```python
from build123d import *

# Parameters (mm, degrees)
SKETCH1_W           = 70
SKETCH1_H           = 70
SKETCH1_R           = 5
BOSS_EXTRUDE1_DEPTH = 5
SKETCH2_W           = 13.5
SKETCH2_H           = 7
SKETCH2_W_2         = 12
BOSS_EXTRUDE2_DEPTH = 20
SKETCH3_R           = 1.75
CUT_EXTRUDE1_DEPTH  = 20
SKETCH4_R           = 4
CUT_EXTRUDE2_DEPTH  = 3
BOSS_EXTRUDE3_START = 1
SKETCH5_R           = 6
SKETCH5_R_2         = 4
BOSS_EXTRUDE3_DEPTH = 1
SKETCH6_R           = 15
CUT_EXTRUDE3_DEPTH  = 83.158383626


with BuildPart() as part:
    # Sketch1 → Boss-Extrude1 (new body)
    with BuildSketch(Plane.XY):
        Rectangle(SKETCH1_W, SKETCH1_H)
        with Locations((0, -14)):
            Circle(SKETCH1_R, mode=Mode.SUBTRACT)
    extrude(amount=BOSS_EXTRUDE1_DEPTH)

    # Sketch2 → Boss-Extrude2 (add)
    with BuildSketch(Plane.XY.offset(5)):
        with Locations((-28.25, -31.5)):
            Rectangle(SKETCH2_W, SKETCH2_H)
        with Locations((28.25, -31.5)):
            Rectangle(SKETCH2_W, SKETCH2_H)
        with Locations((0, -31.5)):
            Rectangle(SKETCH2_W_2, SKETCH2_H)
    extrude(amount=BOSS_EXTRUDE2_DEPTH)

    # Sketch3 → Cut-Extrude1 (cut)
    with BuildSketch(Plane(origin=(0, -28, 0), x_dir=(1, 0, 0), z_dir=(0, 1, 0))):
        with Locations(Location((-28.25, -10, 0), (0, 0, 270))):
            Circle(SKETCH3_R)
        with Locations(Location((28.25, -10, 0), (0, 0, 270))):
            Circle(SKETCH3_R)
        with Locations(Location((0, -20, 0), (0, 0, 270))):
            Circle(SKETCH3_R)
    extrude(amount=-CUT_EXTRUDE1_DEPTH, mode=Mode.SUBTRACT)

    # Sketch4 → Cut-Extrude2 (cut)
    with BuildSketch(Plane.XY.offset(5)):
        with Locations((0, 26)):
            Circle(SKETCH4_R)
    extrude(amount=-CUT_EXTRUDE2_DEPTH, mode=Mode.SUBTRACT)

    # Sketch5 → Boss-Extrude3 (add)
    with BuildSketch(Plane.XY.offset(5).offset(BOSS_EXTRUDE3_START)):
        with Locations((0, 26)):
            Circle(SKETCH5_R)
        with Locations((0, 26)):
            Circle(SKETCH5_R_2, mode=Mode.SUBTRACT)
    extrude(amount=-BOSS_EXTRUDE3_DEPTH)

    # Sketch6 → Cut-Extrude3 (cut, through all)
    with BuildSketch(Plane.XZ.offset(35)):
        with Locations((0, 38.5)):
            Circle(SKETCH6_R)
    extrude(amount=-CUT_EXTRUDE3_DEPTH, mode=Mode.SUBTRACT)


solid = part.part
```
Here's how the part is built. I have some questions about the finished solid (model axes, mm). A direction names the side the tool comes from. Coordinates: 2 decimals unless noted, no trailing zeros. Loops run counter-clockwise (first coordinate to the right, second up) from the corner with the lowest first, then second, coordinate; pieces in that order, holes last. Notation, with made-up numbers: (46, 65.25) -> (87, 65.25) arc R14 cw to (87, 87.25) -> close; hole circle Ø5 at (49, 3). An arc over 180 degrees is marked (long way). Return JSON: item names as keys, results as strings.
1) I need wall thicknesses on line 1 (X direction, y = -30, z = 20); line 2 (X direction, y = -31.75, z = 10); line 3 (X direction, y = -32, z = 18.5). Which ranges of each line are inside material? Lowest first, please. Write a range as from..to.
Results below:
{"line 1": "-35..-21.5, -6..-1.75, 1.75..6, 21.5..35", "line 2": "-35..-30, -26.5..-21.5, -6..6, 21.5..26.5, 30..35", "line 3": "-35..-21.5, -6..-0.9, 0.9..6, 21.5..35"}
2) If we section it at D-D, the plane z = 20: Write out the boundary of the cut face in (x, y), then the cut area to 4 significant figures.
Results below:
{"outline": "(-35, -35) -> (-21.5, -35) -> (-21.5, -28) -> (-35, -28) -> close; (-6, -35) -> (-1.75, -35) -> (-1.75, -28) -> (-6, -28) -> close; (1.75, -35) -> (6, -35) -> (6, -28) -> (1.75, -28) -> close; (21.5, -35) -> (35, -35) -> (35, -28) -> (21.5, -28) -> close", "area": "248.5 mm²"}
3) If we section it at B-B, the plane y = -30: Write out the boundary of the cut face in (x, z).
Results below:
{"outline": "(-35, 0) -> (35, 0) -> (35, 25) -> (21.5, 25) -> (21.5, 5) -> (6, 5) -> (6, 24.75) arc R15 cw to (-6, 24.75) -> (-6, 5) -> (-21.5, 5) -> (-21.5, 25) -> (-35, 25) -> close; hole circle Ø3.5 at (-28.25, 10); hole circle Ø3.5 at (0, 20); hole circle Ø3.5 at (28.25, 10)"}
4) If we section it at C-C, the plane x = 28.25: Write out the boundary of the cut face in (y, z).
Results below:
{"outline": "(-35, 0) -> (35, 0) -> (35, 5) -> (-28, 5) -> (-28, 8.25) -> (-35, 8.25) -> close; (-35, 11.75) -> (-28, 11.75) -> (-28, 25) -> (-35, 25) -> close"}
5) Will these pins go through, and if not, where does the flat tip stop? pin 1 (2 mm diameter, centred on x = 0, z = 20, fed in from +Y); pin 2 (21 mm diameter, centred on x = -13.5, y = 7, fed in from +Z); pin 3 (6.5 mm diameter, centred on x = -1, y = 24.5, fed in from +Z); pin 4 (5 mm diameter, centred on x = -6.5, z = 9, fed in from +Y).
Results below:
{"pin 1": "through", "pin 2": "z = 5", "pin 3": "z = 6", "pin 4": "y = -28"}
6) If we section it at A-A, the plane y = -14: Write out the boundary of the cut face in (x, z), then the cut area to 3 significant figures.
Results below:
{"outline": "(-35, 0) -> (-5, 0) -> (-5, 5) -> (-35, 5) -> close; (5, 0) -> (35, 0) -> (35, 5) -> (5, 5) -> close", "area": "300 mm²"}
7) Thinking about a two-plate mould opening in Z: for faces 4 (the face through (-27.724, -31.451, 11.669)), 5 (the face through (28, -28, 15)), 6 (the face through (-1.42, 22.08, 6)), 7 (the face through (0, 0, 0)), which applies, +Z half, -Z half, draft (parallel to the pull), parting line (faces both ways), or undercut?
Results below:
{"face 4": "undercut", "face 5": "draft", "face 6": "+Z half", "face 7": "-Z half"}
8) For faces 1 (the face through (-28, -28, 15)), 2 (the face through (-1.301, 20.143, 5.507)), 3 (the face through (-21.5, -32, 15)), which set-ups out of +Z, -Z, +X, -X, +Y, -Y let a thin tool reach every point of the face, with its end or its side?
Results below:
{"face 1": "+Z, +X, -X, +Y", "face 2": "+Z", "face 3": "+Z, +Y, -Y"}
